The drawing under review shows one solid part. Ordinate dimensions are in mm from its lowest x, y, z. Give positions to 0.01 mm unless a question says otherwise; leave off trailing zeros. Loops run counter-clockwise (first coordinate to the right, second up) from the corner with the lowest first, then second, coordinate; pieces in that order, holes last. Notation, with made-up numbers: M 20.5,-15 L 76.5,-15 A19 ccw 76.5,-11 Z; hole C 17,58 d4. An arc over 180 degrees is marked long. Put each result on its own line as item: value. Start each with the question number.
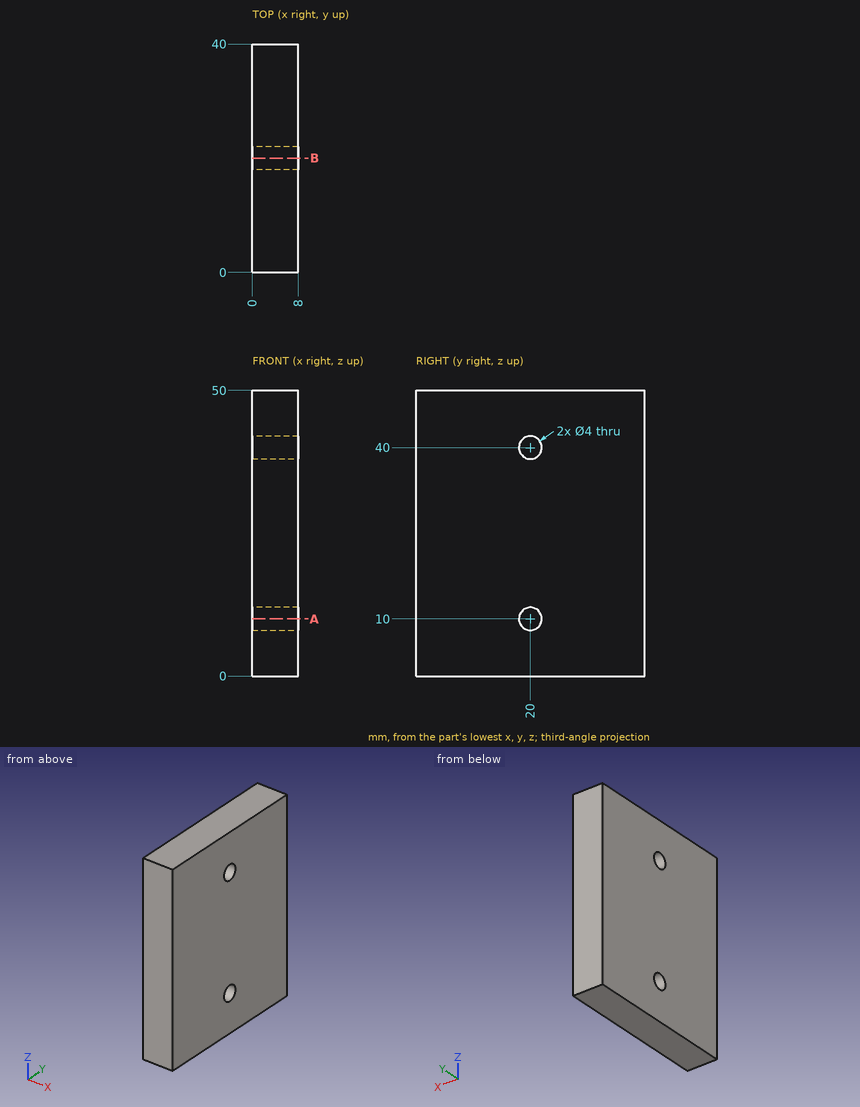
Item 1: Consider section B-B, the plane y = 20. Write out the cut boundary in (x, z), plus the area to 3 significant figures.
Item 2: Clearance check with a flat-ended pin moving along its axis: pin 1 Ø3 at (y, z) = (20, 40) entering from +X (3 decimals). State where the tip first meets the part, or that it passes through.
Item 3: Consider section A-A, the plane z = 10. Write out the cut boundary in (x, y), plus the area to 3 significant figures.
Item 4: To check wall thickness, follow L1, parallel to Z at x = 6.25, y = 21.5; L2, parallel to Y at x = 4.5, z = 10; L3, parallel to Y at x = 7.5, z = 39. State the ranges of each line that lie inside material, in increasing order. Write a range as [from, to].
Report:
1. outline: M 0,0 L 8,0 L 8,8 L 0,8 Z; M 0,12 L 8,12 L 8,38 L 0,38 Z; M 0,42 L 8,42 L 8,50 L 0,50 Z
1. area: 336 mm²
2. pin 1: through
3. outline: M 0,0 L 8,0 L 8,18 L 0,18 Z; M 0,22 L 8,22 L 8,40 L 0,40 Z
3. area: 288 mm²
4. L1: [0, 8.68], [11.32, 38.68], [41.32, 50]
4. L2: [0, 18], [22, 40]
4. L3: [0, 18.27], [21.73, 40]
